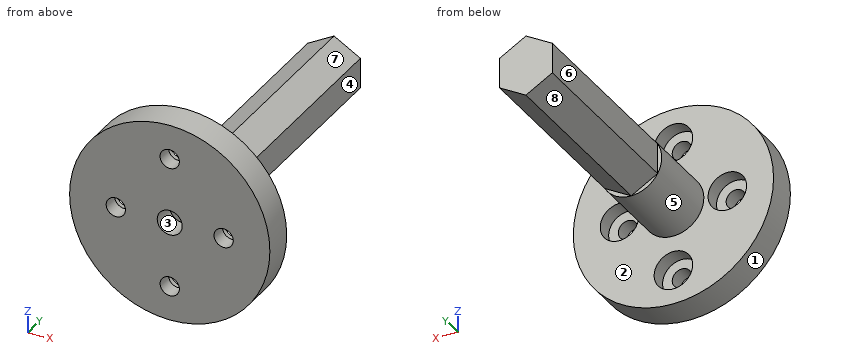
```python
from build123d import *

# Parameters (mm, degrees)
CROQUIS3_R                 = 13
SALIENTE_EXTRUIR1_DEPTH    = 4
CROQUIS4_R                 = 3.95
SALIENTE_EXTRUIR2_DEPTH    = 35
CORTAR_EXTRUIR3_DEPTH      = 44.116122275
CORTAR_EXTRUIR3_DEPTH_BACK = 44.116122275
CROQUIS8_R                 = 1.25
CORTAR_EXTRUIR5_DEPTH      = 40.534794802
CORTAR_EXTRUIR5_DEPTH_BACK = 2
CROQUIS10_R                = 2.5
CROQUIS10_R_2              = 1.25
CROQUIS9_R                 = 1.625
CORTAR_EXTRUIR4_DEPTH      = 3
CROQUIS12_OUTSIDE_W        = 38.72
CROQUIS12_OUTSIDE_H        = 38.72
CORTAR_EXTRUIR7_DEPTH      = 25


with BuildPart() as part:
    # Croquis3 → Saliente-Extruir1 (new body)
    with BuildSketch(Plane(origin=(0, 0, 0), x_dir=(1, 0, 0), z_dir=(0, 1, 0))):
        with Locations(Location((0, 0, 0), (0, 0, 270))):
            Circle(CROQUIS3_R)
    extrude(amount=SALIENTE_EXTRUIR1_DEPTH)

    # Croquis4 → Saliente-Extruir2 (add)
    with BuildSketch(Plane(origin=(0, 4, 0), x_dir=(1, 0, 0), z_dir=(0, 1, 0))):
        with Locations(Location((0, 0, 0), (0, 0, 270))):
            Circle(CROQUIS4_R)
    extrude(amount=SALIENTE_EXTRUIR2_DEPTH)

    # Croquis8 → Cortar-Extruir3 (cut, two sides: drawn at the far end of the back side and taken through both)
    with BuildSketch(Plane.XZ.offset(-CORTAR_EXTRUIR3_DEPTH_BACK)):
        with Locations(Location((0, 8.5, 0), (0, 0, 90))):
            Circle(CROQUIS8_R)
        with Locations(Location((0, -8.5, 0), (0, 0, 90))):
            Circle(CROQUIS8_R)
        with Locations(Location((-7, 0, 0), (0, 0, 90))):
            Circle(CROQUIS8_R)
        with Locations(Location((7, 0, 0), (0, 0, 90))):
            Circle(CROQUIS8_R)
    extrude(amount=CORTAR_EXTRUIR3_DEPTH + CORTAR_EXTRUIR3_DEPTH_BACK, mode=Mode.SUBTRACT)

    # Croquis10 → Cortar-Extruir5 (cut, two sides: drawn at the far end of the back side and taken through both)
    # profile 1 of 4: a face of its own
    with BuildSketch(Plane(origin=(0, 4, 0), x_dir=(1, 0, 0), z_dir=(0, 1, 0)).offset(-CORTAR_EXTRUIR5_DEPTH_BACK)):
        with Locations(Location((0, 8.5, 0), (0, 0, 270))):
            Circle(CROQUIS10_R)
    # profile 2 of 4: a face of its own
    with BuildSketch(Plane(origin=(0, 4, 0), x_dir=(1, 0, 0), z_dir=(0, 1, 0)).offset(-CORTAR_EXTRUIR5_DEPTH_BACK)):
        with Locations(Location((0, -8.5, 0), (0, 0, 270))):
            Circle(CROQUIS10_R)
    # profile 3 of 4: a face of its own
    with BuildSketch(Plane(origin=(0, 4, 0), x_dir=(1, 0, 0), z_dir=(0, 1, 0)).offset(-CORTAR_EXTRUIR5_DEPTH_BACK)):
        with Locations(Location((-7, 0, 0), (0, 0, 270))):
            Circle(CROQUIS10_R)
        with Locations(Location((-7, 0, 0), (0, 0, 270))):
            Circle(CROQUIS10_R_2, mode=Mode.SUBTRACT)
    # profile 4 of 4: a face of its own
    with BuildSketch(Plane(origin=(0, 4, 0), x_dir=(1, 0, 0), z_dir=(0, 1, 0)).offset(-CORTAR_EXTRUIR5_DEPTH_BACK)):
        with Locations(Location((7, 0, 0), (0, 0, 270))):
            Circle(CROQUIS10_R)
        with Locations(Location((7, 0, 0), (0, 0, 270))):
            Circle(CROQUIS10_R_2, mode=Mode.SUBTRACT)
    extrude(amount=CORTAR_EXTRUIR5_DEPTH + CORTAR_EXTRUIR5_DEPTH_BACK, mode=Mode.SUBTRACT)

    # Croquis9 → Cortar-Extruir4 (cut)
    with BuildSketch(Plane(origin=(0, 0, 0), x_dir=(1, 0, 0), z_dir=(0, 1, 0))):
        with Locations(Location((0, 0, 0), (0, 0, 270))):
            Circle(CROQUIS9_R)
    extrude(amount=CORTAR_EXTRUIR4_DEPTH, mode=Mode.SUBTRACT)

    # Croquis12 outside → Cortar-Extruir7 (cut)
    with BuildSketch(Plane(origin=(0, 39, 0), x_dir=(1, 0, 0), z_dir=(0, 1, 0))):
        Rectangle(CROQUIS12_OUTSIDE_W, CROQUIS12_OUTSIDE_H)
        Polygon((0, 3.95), (-3.420800345, 1.975), (-3.420800345, -1.975), (0, -3.95), (3.420800345, -1.975), (3.420800345, 1.975), align=None, mode=Mode.SUBTRACT)
    extrude(amount=-CORTAR_EXTRUIR7_DEPTH, mode=Mode.SUBTRACT)


solid = part.part
```
Input: part model. Units: mm. Frame: model coordinates. Face numbers are marked on the shaded views. A direction names the side the tool comes from. Round coordinates to 2 decimals unless told otherwise and drop trailing zeros. Loops run counter-clockwise (first coordinate to the right, second up) from the corner with the lowest first, then second, coordinate; pieces in that order, holes last. Notation, with made-up numbers: M 39,-19 L 62,-19 A24 cw 62,-3 Z; hole C -33,52 d7. An arc over 180 degrees is marked long. Answer in a Markdown table with one row per item. Add a question column.
1. Ray query, probe 1 along X at (y, z) = (1.25, 0) (3 decimals); probe 2 along X at (y, z) = (2.2, 0) (3 decimals); probe 3 along Y at (x, z) = (2.25, 7.25). Return the intervals inside material, ascending.
2. Contact query for flat-ended pins moving along their axis: pin 1 (1.2 mm diameter, centred on y = 25, z = 0.5, fed in from +X); pin 2 (10 mm diameter, centred on y = 28, z = 6.5, fed in from -X); pin 3 (1 mm diameter, centred on x = -0.5, z = 0, fed in from -Y); pin 4 (2 mm diameter, centred on x = 0, z = 8.5, fed in from -Y). Output: stop coordinate, or through.
3. Set-up query: the marked faces 4, 5, 6, 7 and 8. Return all of +Z, -Z, +X, -X, +Y, -Y with unobstructed straight access to the full face (end or side cutting, diameter ignored); none if empty.
4. Section A-A (z = 0). Give the number of separate pieces and of enclosed holes in the cut face, and give its area (3 significant figures).
5. Section B-B (x = -7). Output: boundary loops of the cut face in (y, z).
6. Mould query, pull axis Z, two halves, no side actions, for the marked faces 1, 2 and 3. Classes: released by +Z, released by -Z, zero draft, split by the parting line, or undercut.
7. Section C-C (y = 22.5). Output: boundary loops of the cut face in (x, z) (3 decimals).
Values follow:
| question | item | result |
|---|---|---|
| 1 | probe 1 | -13 to -8.25, -5.75 to -1.625, 1.625 to 5.75, 8.25 to 13 |
| 1 | probe 2 | -13 to -9.5, -4.5 to -1.625, 1.625 to 4.5, 9.5 to 13 |
| 1 | probe 3 | 0 to 4 |
| 2 | pin 1 | x = 3.42 |
| 2 | pin 2 | x = -3.42 |
| 2 | pin 3 | y = 3 |
| 2 | pin 4 | through |
| 3 | face 4 | +Z, -Z, +X, +Y |
| 3 | face 5 | +Y |
| 3 | face 6 | +Z, -Z, -X, +Y |
| 3 | face 7 | +Z, +X, +Y |
| 3 | face 8 | -Z, -X, +Y |
| 4 | separate pieces | 3 |
| 4 | enclosed holes | 0 |
| 4 | area | 314 mm^2 |
| 5 | outline | M 0,-10.95 L 4,-10.95 L 4,-2.5 L 2,-2.5 L 2,-1.25 L 0,-1.25 Z; M 0,1.25 L 2,1.25 L 2,2.5 L 4,2.5 L 4,10.95 L 0,10.95 Z |
| 6 | face 1 | split by the parting line |
| 6 | face 2 | zero draft |
| 6 | face 3 | undercut |
| 7 | outline | M -3.421,-1.975 L 0,-3.95 L 3.421,-1.975 L 3.421,1.975 L 0,3.95 L -3.421,1.975 Z |
